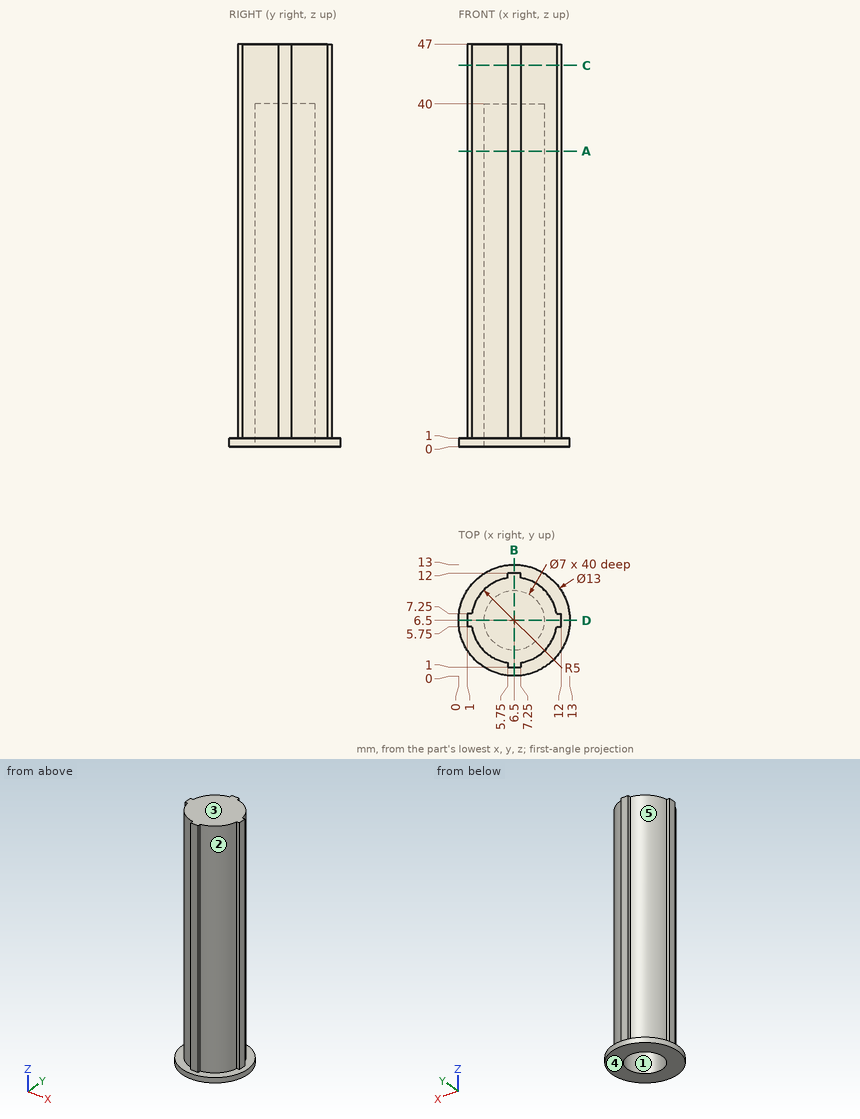
Job drawing, mm, ordinate dimensions from the low corner. One solid piece. A direction names the side the tool comes from. Round coordinates to 2 decimals unless told otherwise and drop trailing zeros. Loops run counter-clockwise (first coordinate to the right, second up) from the corner with the lowest first, then second, coordinate; pieces in that order, holes last. Notation, with made-up numbers: M -25.5,-4 L 25.5,-4 A18 cw 25.5,0 Z; hole C 76.5,61.25 d9. An arc over 180 degrees is marked long. Answer as CSV lines item,"result".
1. Wall check: probe 1 along Y at (x, z) = (6.5, 28.5); probe 2 along Y at (x, z) = (1.25, 15). Give the ranges that are in metal, low to high. Write a range as [from, to].
Resolved:
probe 1,"y = [1, 3], [10, 12]"
probe 2,"y = [5.75, 7.25]"
2. 3-axis set-ups, long thin cutter, end or side, ignore diameter. For the marked faces 4 and 5: which of +Z, -Z, +X, -X, +Y, -Y reach the whole face in a straight line?
Resolved:
face 4,"-Z, +X, -X, +Y, -Y"
face 5,"+Z, -X, +Y"
3. Cut at B-B on x = 6.5. Write the cut outline in (y, z), then the cut area to 3 significant figures.
Resolved:
outline,"M 0,0 L 3,0 L 3,40 L 10,40 L 10,0 L 13,0 L 13,1 L 12,1 L 12,47 L 1,47 L 1,1 L 0,1 Z"
area,"239 mm²"
4. Cut at A-A on z = 34.5. Write the cut outline in (x, y), then the cut area to 3 significant figures.
Resolved:
outline,"M 1,5.75 L 1.56,5.75 A5 ccw 5.75,1.56 L 5.75,1 L 7.25,1 L 7.25,1.56 A5 ccw 11.44,5.75 L 12,5.75 L 12,7.25 L 11.44,7.25 A5 ccw 7.25,11.44 L 7.25,12 L 5.75,12 L 5.75,11.44 A5 ccw 1.56,7.25 L 1,7.25 Z; hole C 6.5,6.5 d7"
area,"43.2 mm²"
5. Two-plate mould, pull along Y, no slides. Class the marked faces 1, 2 and 3: released by +Y, released by -Y, zero draft, split by the parting line, or undercut.
Resolved:
face 1,"undercut"
face 2,"released by -Y"
face 3,"zero draft"
6. Flat gauge pins, fed straight in: P1, Ø1.5, axis at x = 6.5, z = 34.5, coming from the +Y side; P2, Ø3, axis at y = 9.5, z = 5.5, coming from the +X side; P3, Ø1, axis at y = 6.5, z = 39.5, coming from the -X side. Where does each tip first touch, or does it go through?
Resolved:
P1,"stops at y = 12"
P2,"stops at x = 11.27"
P3,"stops at x = 1"
7. Cut at C-C on z = 44.5. Write the cut outline in (x, y), then the cut area to 4 significant figures.
Resolved:
outline,"M 1,5.75 L 1.56,5.75 A5 ccw 5.75,1.56 L 5.75,1 L 7.25,1 L 7.25,1.56 A5 ccw 11.44,5.75 L 12,5.75 L 12,7.25 L 11.44,7.25 A5 ccw 7.25,11.44 L 7.25,12 L 5.75,12 L 5.75,11.44 A5 ccw 1.56,7.25 L 1,7.25 Z"
area,"81.65 mm²"
